from build123d import *

# Parameters (mm, degrees)
F0_W        = 114.2217256129
F0_H        = 42.490478605
F1_DEPTH    = 12.7
F2_W        = 93.6551205814
F2_H        = 25.7396511734
F3_DEPTH    = 2.54
F4_R        = 5.08
F5_SIZE     = 5.08
F6_T1_DEPTH = 39.0415311919
F7_R        = 5.08


# Not quite as in the source:
# - a fillet or chamfer that OpenCascade refuses, or shapes differently, is made with other operations: its cross-section is extruded or revolved along the edge and cut away or added


with BuildPart() as f1:
    # F0 (on Right) → F1 (new body)
    with BuildSketch(Plane.YZ):
        with Locations((10.7826646417, 2.6869159192)):
            Rectangle(F0_W, F0_H)
    extrude(amount=F1_DEPTH)

    # F2 (on face) → F3 (join)
    with BuildSketch(Plane(origin=(0, 0, 0), x_dir=(0, -1, 0), z_dir=(-1, 0, 0))):
        with Locations((-10.6990095228, 3.1011626124)):
            Rectangle(F2_W, F2_H)
    extrude(amount=F3_DEPTH)

    # F4
    f4_edges = [f1.edges().sort_by_distance(p)[0] for p in [
        (-1.27, 57.52657, 15.970988),
        (-1.27, 57.52657, -9.768663),
        (-1.27, -36.128551, -9.768663),
        (-1.27, -36.128551, 15.970988),
    ]]
    fillet(f4_edges, radius=F4_R)

    # F5
    f5_edges = [f1.edges().sort_by_distance(p)[0] for p in [
        (6.35, 67.893527, 23.932155),
        (6.35, -46.328198, 23.932155),
        (6.35, 67.893527, -18.558323),
        (6.35, -46.328198, -18.558323),
    ]]
    chamfer(f5_edges, length=F5_SIZE)

    # F6: chamfer of 5.08 on 8 edges, made by hand

    # F6_s2 → F6_t1 (cut)
    with BuildSketch(Plane.YZ.offset(-13.170765596)):
        Polygon((64.3014249997, 22.4442576701), (67.8935274482, 13.7721552217), (67.8935274482, 18.8521552217), align=None)
        Polygon((57.7335274482, 23.9321552217), (66.4056298966, 20.3400527733), (62.8135274482, 23.9321552217), align=None)
        Polygon((66.4056298966, -14.9662209349), (57.7335274482, -18.5583233833), (62.8135274482, -18.5583233833), align=None)
        Polygon((67.8935274482, -8.3983233833), (64.3014249997, -17.0704258318), (67.8935274482, -13.4783233833), align=None)
        Polygon((-44.8403006131, -14.9662209349), (-36.1681981647, -18.5583233833), (-41.2481981647, -18.5583233833), align=None)
        Polygon((-46.3281981647, -8.3983233833), (-42.7360957163, -17.0704258318), (-46.3281981647, -13.4783233833), align=None)
        Polygon((-42.7360957163, 22.4442576701), (-46.3281981647, 13.7721552217), (-46.3281981647, 18.8521552217), align=None)
        Polygon((-36.1681981647, 23.9321552217), (-44.8403006131, 20.3400527733), (-41.2481981647, 23.9321552217), align=None)
    extrude(amount=F6_T1_DEPTH, mode=Mode.SUBTRACT)

    # F7
    f7_edges = [f1.edges().sort_by_distance(p)[0] for p in [
        (6.35, -43.352403, -15.582528),
        (6.35, -46.328198, -8.398323),
        (6.35, -36.168198, -18.558323),
        (6.35, -46.328198, 13.772155),
        (6.35, -43.352403, 20.95636),
        (6.35, -36.168198, 23.932155),
        (6.35, 57.733527, 23.932155),
        (6.35, 64.917732, 20.95636),
        (6.35, 67.893527, 13.772155),
        (6.35, 67.893527, -8.398323),
        (6.35, 64.917732, -15.582528),
        (6.35, 57.733527, -18.558323),
    ]]
    fillet(f7_edges, radius=F7_R)


solid = f1.part
CAD build for the part. Positions are in the model's coordinates, mm. A direction names the side the tool comes from. Coordinates: 2 decimals unless noted, no trailing zeros. Loops run counter-clockwise (first coordinate to the right, second up) from the corner with the lowest first, then second, coordinate; pieces in that order, holes last. Notation, with made-up numbers: (53.5, 48) - (86.5, 48) arc R24 ccw to (86.5, 71) - close; hole circle Ø2 at (81.5, -10.5). An arc over 180 degrees is marked (long way). Write item = value, one per line. Start each with the question number.
Q1. Cut at A-A, the plane y = 28.5. List the corners of the cut face in (x, z).
Q2. Drill centre lines: L1, parallel to X at y = 30, z = -16; L2, parallel to Z at x = -2, y = -5; L3, parallel to Z at x = 4, y = -40.5. Where is each one in solid material? Low to high.
Q3. Cut at B-B, the plane z = -1.5. List the corners of the cut face in (x, y).
Q4. Flat gauge pins, fed straight in: pin 1 Ø2 at (x, z) = (-2, 5.5) entering from +Y; pin 2 Ø8 at (x, z) = (2.5, 16) entering from +Y; pin 3 Ø4 at (y, z) = (-19, 19.5) entering from -X; pin 4 Ø0.8 at (x, z) = (-1.5, 0.5) entering from -Y. Where does each tip first touch, or does it go through?
Q5. Cut at D-D, the plane z = 17.5. List the corners of the cut face in (x, y).
Q6. Pull direction Z, two halves, no side cores. Call faces 6 (the cylindrical face through (-1.288, -34.601, 14.522)), 7 (the flat face through (12.7, 10, 3)), 8 (the flat face through (-1, 11, -9.769)): pulls with the +Z half, pulls with the -Z half, needs draft (parallel to the pull), parting line crosses it, or undercut.
Q7. Cut at C-C, the plane x = 7.25. List the corners of the cut face in (y, z), then the cut area to 3 significant figures.
Q8. Which spindle directions (+Z, -Z, +X, -X, +Y, -Y) get a long thin tool onto all of the face, cutting with end or side? Do faces 1 (the flat face through (-1, 11, 15.971)), 2 (the cylindrical face through (-1.29, 56.08, 14.44)), 3 (the cylindrical face through (-1.29, 56.08, -8.24)), 4 (the flat face through (-1, 57.527, 3)), 5 (the flat face through (6.261, 60.79, 22.666)). Say none if no direction does.
Computed:
q1.outline = (-2.54, -9.77) - (0, -9.77) - (0, -18.56) - (12.7, -18.56) - (12.7, 23.93) - (0, 23.93) - (0, 15.97) - (-2.54, 15.97) - close
q2.L1 = 0 to 12.7
q2.L2 = -9.77 to 15.97
q2.L3 = -16.76 to 22.14
q3.outline = (-2.54, -36.13) - (0, -36.13) - (0, -46.33) - (12.7, -46.33) - (12.7, 67.89) - (0, 67.89) - (0, 57.53) - (-2.54, 57.53) - close
q4.pin_1 = 57.53
q4.pin_2 = 67.89
q4.pin_3 = 0
q4.pin_4 = -36.13
q5.outline = (0, -44.78) - (12.7, -44.78) - (12.7, 66.35) - (0, 66.35) - close
q6.face_6 = pulls with the +Z half
q6.face_7 = needs draft
q6.face_8 = pulls with the -Z half
q7.outline = (-46.33, -7.39) arc R5.08 ccw to (-45.94, -9.33) - (-44.16, -13.64) arc R5.08 ccw to (-41.41, -16.39) - (-37.1, -18.17) arc R5.08 ccw to (-35.16, -18.56) - (56.72, -18.56) arc R5.08 ccw to (58.67, -18.17) - (62.97, -16.39) arc R5.08 ccw to (65.72, -13.64) - (67.51, -9.33) arc R5.08 ccw to (67.89, -7.39) - (67.89, 12.76) arc R5.08 ccw to (67.51, 14.71) - (65.72, 19.01) arc R5.08 ccw to (62.97, 21.76) - (58.67, 23.55) arc R5.08 ccw to (56.72, 23.93) - (-35.16, 23.93) arc R5.08 ccw to (-37.1, 23.55) - (-41.41, 21.76) arc R5.08 ccw to (-44.16, 19.01) - (-45.94, 14.71) arc R5.08 ccw to (-46.33, 12.76) - close
q7.area = 4,730 mm²
q8.face_1 = +Z, -X, +Y, -Y
q8.face_2 = +Z, -X, +Y
q8.face_3 = -Z, -X, +Y
q8.face_4 = +Z, -Z, -X, +Y
q8.face_5 = +Z, +X, -X, +Y
